from build123d import *

# Parameters (mm, degrees)
SALIENTE_EXTRUIR1_DEPTH = 400
CROQUIS2_R              = 1.5
CORTAR_EXTRUIR1_DEPTH   = 10
CROQUIS3_R              = 1.5875
CORTAR_EXTRUIR2_DEPTH   = 14.7


with BuildPart() as part:
    # Croquis1 → Saliente-Extruir1 (new body, symmetric)
    with BuildSketch(Plane.XY):
        Polygon((0, 13.7), (12.7, 13.7), (12.7, 1), (25.4, 1), (25.4, 0), (-25.4, 0), (-25.4, 1), (-12.7, 1), (-12.7, 13.7), align=None)
        Polygon((0, 12.7), (-11.7, 12.7), (-11.7, 1), (11.7, 1), (11.7, 12.7), align=None, mode=Mode.SUBTRACT)
    extrude(amount=SALIENTE_EXTRUIR1_DEPTH, both=True)

    # Croquis2 → Cortar-Extruir1 (cut)
    with BuildSketch(Plane.XZ):
        with Locations((-20, 395)):
            Circle(CROQUIS2_R)
        with Locations((20, 395)):
            Circle(CROQUIS2_R)
        with Locations((20, -395)):
            Circle(CROQUIS2_R)
        with Locations((-20, -395)):
            Circle(CROQUIS2_R)
    extrude(amount=-CORTAR_EXTRUIR1_DEPTH, mode=Mode.SUBTRACT)

    # Croquis3 → Cortar-Extruir2 (cut, through all)
    with BuildSketch(Plane.XZ):
        Circle(CROQUIS3_R)
        with Locations((0, 50)):
            Circle(CROQUIS3_R)
        with Locations((0, 100)):
            Circle(CROQUIS3_R)
        with Locations((0, 150)):
            Circle(CROQUIS3_R)
        with Locations((0, 200)):
            Circle(CROQUIS3_R)
        with Locations((0, 250)):
            Circle(CROQUIS3_R)
        with Locations((0, 300)):
            Circle(CROQUIS3_R)
        with Locations((0, 350)):
            Circle(CROQUIS3_R)
        with Locations((0, -50)):
            Circle(CROQUIS3_R)
        with Locations((0, -100)):
            Circle(CROQUIS3_R)
        with Locations((0, -150)):
            Circle(CROQUIS3_R)
        with Locations((0, -200)):
            Circle(CROQUIS3_R)
        with Locations((0, -250)):
            Circle(CROQUIS3_R)
        with Locations((0, -300)):
            Circle(CROQUIS3_R)
        with Locations((0, -350)):
            Circle(CROQUIS3_R)
    extrude(amount=-CORTAR_EXTRUIR2_DEPTH, mode=Mode.SUBTRACT)


solid = part.part
Geometry: final body of the model. Coordinates: model frame, mm. A direction names the side the tool comes from. Coordinates: 2 decimals unless noted, no trailing zeros. Loops run counter-clockwise (first coordinate to the right, second up) from the corner with the lowest first, then second, coordinate; pieces in that order, holes last. Notation, with made-up numbers: M -32,54 L 19,54 A24 ccw 19,65 Z; hole C -37.5,12.5 d1. An arc over 180 degrees is marked long. One line per item, written item: value. Start each with the question number.
1) Pin query (flat end, axial travel): P1, Ø8, axis at y = 1.5, z = -114.5, coming from the -X side; P2, Ø12, axis at x = -19, z = 73, coming from the +Y side; P3, Ø3, axis at x = 0, z = -350, coming from the +Y side; P4, Ø6, axis at y = 10.5, z = 178.5, coming from the -X side. Return the tip coordinate at first contact, or that it passes through.
2) Cut plane B-B (y = 3.75). Return loops of the section in (x, z).
3) Material intervals for L1, parallel to X at y = 8.25, z = 54; L2, parallel to X at y = 0.6, z = -395; L3, parallel to X at y = 13.3, z = 250, sorted ascending. Write a range as from..to.
4) Draft query along X for faces 1 (the flat face through (12.7, 7, 6)), 2 (the flat face through (19, 1, 6)), 3 (the flat face through (0, 12.7, 6)), 4 (the flat face through (-12.7, 7, 6)). Return one class per face: released by +X, released by -X, zero draft, split by the parting line, or undercut.
5) Cut plane A-A (z = 126). Return loops of the section in (x, y), then the cut area to 3 significant figures.
6) Reachability of faces 5 (the flat face through (-19, 1, 6)), 6 (the flat face through (0, 13.7, 6)), 7 (the flat face through (0, 1, 6)) from +Z, -Z, +X, -X, +Y, -Y: full face, straight path, thin tool, end or side. Return the list, or none.
Evaluation:
1. P1: x = -25.4
1. P2: y = 1
1. P3: through
1. P4: x = -12.7
2. outline: M -12.7,-400 L -11.7,-400 L -11.7,400 L -12.7,400 Z; M 11.7,-400 L 12.7,-400 L 12.7,400 L 11.7,400 Z
3. L1: -12.7..-11.7, 11.7..12.7
3. L2: -25.4..-21.5, -18.5..18.5, 21.5..25.4
3. L3: -12.7..-1.59, 1.59..12.7
4. face 1: released by +X
4. face 2: zero draft
4. face 3: undercut
4. face 4: released by -X
5. outline: M -25.4,0 L 25.4,0 L 25.4,1 L 12.7,1 L 12.7,13.7 L -12.7,13.7 L -12.7,1 L -25.4,1 Z; hole M -11.7,1 L 11.7,1 L 11.7,12.7 L -11.7,12.7 Z
5. area: 99.6 mm^2
6. face 5: +Z, -Z, -X, +Y
6. face 6: +Z, -Z, +X, -X, +Y
6. face 7: +Z, -Z
